CAD build for the part. Positions are in the model's coordinates, mm. A direction names the side the tool comes from. Round coordinates to 2 decimals unless told otherwise and drop trailing zeros. Loops run counter-clockwise (first coordinate to the right, second up) from the corner with the lowest first, then second, coordinate; pieces in that order, holes last.
from build123d import *

# Parameters (mm, degrees)
SKETCH1_R           = 8.255
SKETCH1_R_2         = 6.985
BOSS_EXTRUDE1_DEPTH = 19.05
SKETCH2_R           = 11.43
SKETCH2_R_2         = 8.255
BOSS_EXTRUDE2_DEPTH = 3.81
BOSS_EXTRUDE3_START = 12.7
SKETCH3_R           = 8.255
SKETCH3_R_2         = 6.985
BOSS_EXTRUDE3_DEPTH = 12.7


with BuildPart() as part:
    # Sketch1 → Boss-Extrude1 (new body)
    with BuildSketch(Plane.XY):
        with Locations(Location((0, 0, 0), (0, 0, 180))):
            Circle(SKETCH1_R)
        with Locations(Location((0, 0, 0), (0, 0, 180))):
            Circle(SKETCH1_R_2, mode=Mode.SUBTRACT)
    extrude(amount=BOSS_EXTRUDE1_DEPTH)

    # Sketch2 → Boss-Extrude2 (add)
    with BuildSketch(Plane.XY):
        with Locations(Location((0, 0, 0), (0, 0, 180))):
            Circle(SKETCH2_R)
        with Locations(Location((0, 0, 0), (0, 0, 180))):
            Circle(SKETCH2_R_2, mode=Mode.SUBTRACT)
    boss_extrude2 = extrude(amount=BOSS_EXTRUDE2_DEPTH)

    # Sketch3 → Boss-Extrude3 (add)
    with BuildSketch(Plane(origin=(0, 0, 0), x_dir=(-1, 0, 0), z_dir=(0, 0, -1)).offset(BOSS_EXTRUDE3_START)):
        Circle(SKETCH3_R)
        Circle(SKETCH3_R_2, mode=Mode.SUBTRACT)
    boss_extrude3 = extrude(amount=-BOSS_EXTRUDE3_DEPTH)

    # Mirror1: Boss-Extrude2 across plane
    add(boss_extrude2.mirror(Plane(origin=(0, 0, 9.525), x_dir=(1, 0, 0), z_dir=(0, 0, -1))))

    # Mirror2: Boss-Extrude3 across plane
    add(boss_extrude3.mirror(Plane(origin=(0, 0, 9.525), x_dir=(1, 0, 0), z_dir=(0, 0, -1))))


solid = part.part
Item 1: Cut at A-A (x = 0). List the corners of the cut face in (y, z) (3 decimals), plus the area to 3 significant figures.
Verdict:
outline: (-11.43, 0) - (-8.255, 0) - (-8.255, -12.7) - (-6.985, -12.7) - (-6.985, 31.75) - (-8.255, 31.75) - (-8.255, 19.05) - (-11.43, 19.05) - (-11.43, 15.24) - (-8.255, 15.24) - (-8.255, 3.81) - (-11.43, 3.81) - close; (6.985, -12.7) - (8.255, -12.7) - (8.255, 0) - (11.43, 0) - (11.43, 3.81) - (8.255, 3.81) - (8.255, 15.24) - (11.43, 15.24) - (11.43, 19.05) - (8.255, 19.05) - (8.255, 31.75) - (6.985, 31.75) - close
area: 161 mm2
Item 2: Mould opens along Z. For faces 1 (the flat face through (-3, 8, 0)), 2 (the cylindrical face through (9.07, 6.955, 17.172)), 3 (the flat face through (-3, 8, 3.81)), 4 (the flat face through (7, 2, 31.75)) say: released by +Z, released by -Z, zero draft, split by the parting line, or undercut.
Verdict:
face 1: released by -Z
face 2: zero draft
face 3: undercut
face 4: released by +Z
Item 3: Flat gauge pins, fed straight in: P1, Ø6, axis at x = -3, y = 3.5, coming from the -Z side; P2, Ø2, axis at y = -2.5, z = 14.5, coming from the -X side; P3, Ø1, axis at y = 4, z = 14.5, coming from the +X side; P4, Ø5, axis at x = -6, z = 14, coming from the +Y side. Where does each tip first touch, or does it go through?
Verdict:
P1: stops at z = -12.7
P2: stops at x = -11.28
P3: stops at x = 7.48
P4: stops at y = 10.77
Item 4: Cut at C-C (z = -7.5). List the corners of the cut face in (x, y) (3 decimals), plus the area to 3 significant figures.
Verdict:
outline: circle Ø16.51 at (0, 0); hole circle Ø13.97 at (0, 0)
area: 60.8 mm2
Item 5: Wall check: L1, parallel to Z at x = 0.5, y = 9.5; L2, parallel to Y at x = 0, z = 12.25 (3 decimals); L3, parallel to Y at x = 6, z = 8. Give the ranges that are in metal, low to high.
Verdict:
L1: z = 0 to 3.81, 15.24 to 19.05
L2: y = -8.255 to -6.985, 6.985 to 8.255
L3: y = -5.67 to -3.58, 3.58 to 5.67
Item 6: Cut at D-D (y = 10.25). List the corners of the cut face in (x, z), plus the area to 3 significant figures.
Verdict:
outline: (-5.06, 0) - (5.06, 0) - (5.06, 3.81) - (-5.06, 3.81) - close; (-5.06, 15.24) - (5.06, 15.24) - (5.06, 19.05) - (-5.06, 19.05) - close
area: 77.1 mm2
Item 7: 3-axis set-ups, long thin cutter, end or side, ignore diameter. For faces 5 (the cylindrical face through (-7.874, 2.48, -6.439)), 6 (the cylindrical face through (-7.874, 2.48, 25.489)), 7 (the flat face through (7, 2, -12.7)), 8 (the cylindrical face through (-7.874, -2.48, 9.445)): which of +Z, -Z, +X, -X, +Y, -Y reach the whole face in a straight line?
Verdict:
face 5: -Z
face 6: +Z
face 7: -Z, +X, -X, +Y, -Y
face 8: none
